from build123d import *

# Parameters (mm, degrees)
SKETCH1_W                                  = 111
SKETCH1_H                                  = 18
BASEPLATE_DEPTH                            = 600
SKETCH2_W                                  = 18
SKETCH2_H                                  = 600
SIDE_RAIL_DEPTH                            = 50
SKETCH3_W                                  = 30.5
SKETCH3_H                                  = 600
KEEPER_RAIL_DEPTH                          = 18
SKETCH5_W                                  = 111
SKETCH5_H                                  = 50
LAP_JOINT_CUTOUT_DEPTH                     = 18
LAP_JOINT_BOLT_HOLE_PATTERN_D              = 6.6
LAP_JOINT_BOLT_HOLE_PATTERN_DEPTH          = 57
LAP_JOINT_BOLT_HOLE_PATTERN_TIP            = 1.982840043
FIXED_BEARING_BLOCK_BOLT_CLEARANCE_HOLES_D = 6.6
CROSS_DOWEL_BOLT_CLEARANCE_HOLES_D         = 10


with BuildPart() as part:
    # Sketch1 → baseplate (new body)
    with BuildSketch(Plane.XY):
        with Locations((55.5, 9)):
            Rectangle(SKETCH1_W, SKETCH1_H)
    extrude(amount=BASEPLATE_DEPTH)

    # Sketch2 → side_rail (add)
    with BuildSketch(Plane(origin=(0, 18, 0), x_dir=(1, 0, 0), z_dir=(0, 1, 0))):
        with Locations((9, -300)):
            Rectangle(SKETCH2_W, SKETCH2_H)
    side_rail = extrude(amount=SIDE_RAIL_DEPTH)

    # Sketch3 → keeper rail (add)
    with BuildSketch(Plane(origin=(0, 68, 0), x_dir=(1, 0, 0), z_dir=(0, 1, 0))):
        with Locations((15.25, -300)):
            Rectangle(SKETCH3_W, SKETCH3_H)
    keeper_rail = extrude(amount=KEEPER_RAIL_DEPTH)

    # mirror rails: side_rail, keeper rail across plane
    add(side_rail.mirror(Plane.ZY.offset(-55.5)))
    add(keeper_rail.mirror(Plane.ZY.offset(-55.5)))

    # Sketch5 → lap joint cutout (cut)
    with BuildSketch(Plane.XZ):
        with Locations((55.5, 25)):
            Rectangle(SKETCH5_W, SKETCH5_H)
    extrude(amount=-LAP_JOINT_CUTOUT_DEPTH, mode=Mode.SUBTRACT)

    # lap joint bolt hole pattern
    with Locations(Plane(origin=(0, 18, 0), x_dir=(-1, 0, 0), z_dir=(0, -1, 0))):
        with Locations((-102, -10), (-9, -40), (-102, -40), (-9, -10)):
            Hole(LAP_JOINT_BOLT_HOLE_PATTERN_D / 2, depth=LAP_JOINT_BOLT_HOLE_PATTERN_DEPTH)
            with Locations((0, 0, -(LAP_JOINT_BOLT_HOLE_PATTERN_DEPTH + LAP_JOINT_BOLT_HOLE_PATTERN_TIP / 2))):  # 118° drill point
                Cone(0, LAP_JOINT_BOLT_HOLE_PATTERN_D / 2, LAP_JOINT_BOLT_HOLE_PATTERN_TIP, mode=Mode.SUBTRACT)

    # fixed bearing block bolt clearance holes (through all)
    with Locations(Plane(origin=(0, 18, 0), x_dir=(1, 0, 0), z_dir=(0, 1, 0))):
        with Locations((37.5, -535), (73.5, -535)):
            Hole(FIXED_BEARING_BLOCK_BOLT_CLEARANCE_HOLES_D / 2)

    # cross dowel bolt clearance holes (through all)
    with Locations(Plane(origin=(111, 0, 0), x_dir=(0, 0, -1), z_dir=(1, 0, 0))):
        with Locations((-40, 60), (-10, 60)):
            Hole(CROSS_DOWEL_BOLT_CLEARANCE_HOLES_D / 2)


solid = part.part
Part model, mm, in its own coordinate system. A direction names the side the tool comes from. Round coordinates to 2 decimals unless told otherwise and drop trailing zeros. Write each loop counter-clockwise with the first axis right and the second up, starting at its lowest first coordinate (ties: lowest second). Pieces come first, ordered by that corner, then holes. Notation, with made-up numbers: M -29.75,67.5 L 8.25,67.5 A16 ccw 8.25,98.5 Z; hole C -33,88 d2. An arc over 180 degrees is marked long. Return JSON: item names as keys, results as strings. Group by question number.
(1) Which spindle directions (+Z, -Z, +X, -X, +Y, -Y) get a long thin tool onto all of the face, cutting with end or side? Do faces 1 (the face through (102, 18, 25)), 2 (the face through (9, 63, 36)), 3 (the face through (111, 42, 304)), 4 (the face through (80.5, 77, 304)), 5 (the face through (18, 43, 304)). Say none if no direction does.
(2) Drill centre lines: probe 1 along X at (y, z) = (40, 10); probe 2 along Z at (x, y) = (102, 68.5); probe 3 along X at (y, z) = (7, 535). Where is each one in solid material? Low to high.
(3) Two-plate mould, pull along Y, no slides. Class faces 6 (the face through (12, 59, 0)), 7 (the face through (96, 86, 296)), 8 (the face through (102, 63, 36)): +Y half, -Y half, draft (parallel to the pull), parting line (faces both ways), or undercut.
(4) Pin check, flat tips, straight feed: pin 1 Ø3 at (x, z) = (46.5, 363) entering from +Y; pin 2 Ø12 at (x, y) = (62, 9) entering from -Z; pin 3 Ø8.5 at (x, z) = (102, 10) entering from -Y. Stop position of each tip, or through.
(5) Saw through at B-B on z = 341.5. Write the cut outline in (x, y).
(6) Saw through at A-A on y = 26.5. Write the cut outline in (x, z), then the cut area to 3 significant figures.
Returned:
{
 "1": {"face 1": "-Z, +X, -X, -Y", "face 2": "+X, -X", "face 3": "+Z, -Z, +X, +Y, -Y", "face 4": "+Z, -Z, +Y", "face 5": "+Z, -Z"},
 "2": {"probe 1": "0 to 5.7, 12.3 to 18, 93 to 98.7, 105.3 to 111", "probe 2": "0 to 6.7, 13.3 to 36.7, 43.3 to 600", "probe 3": "0 to 34.2, 40.8 to 70.2, 76.8 to 111"},
 "3": {"face 6": "draft", "face 7": "+Y half", "face 8": "undercut"},
 "4": {"pin 1": "y = 18", "pin 2": "z = 50", "pin 3": "y = 18"},
 "5": {"outline": "M 0,0 L 111,0 L 111,86 L 80.5,86 L 80.5,68 L 93,68 L 93,18 L 18,18 L 18,68 L 30.5,68 L 30.5,86 L 0,86 Z"},
 "6": {"outline": "M 0,0 L 18,0 L 18,600 L 0,600 Z; M 93,0 L 111,0 L 111,600 L 93,600 Z; hole C 9,10 d6.6; hole C 9,40 d6.6; hole C 102,10 d6.6; hole C 102,40 d6.6", "area": "21,500 mm²"}
}
